Design review of the part built by this model. Coordinates are the model's own, in mm. A direction names the side the tool comes from. Coordinates: 2 decimals unless noted, no trailing zeros. Write each loop counter-clockwise with the first axis right and the second up, starting at its lowest first coordinate (ties: lowest second). Pieces come first, ordered by that corner, then holes. Notation, with made-up numbers: (33.5, 85) -> (56.5, 85) arc R15 cw to (56.5, 102) -> close; hole circle Ø1 at (22, 80). An arc over 180 degrees is marked (long way). Write item = value, one per line. Start each with the question number.
```python
from build123d import *

# Parameters (mm, degrees)
SKIZZE1_W                            = 51
SKIZZE1_H                            = 26
SKIZZE1_R                            = 9
AUFSATZ_LINEAR_AUSTRAGEN1_DEPTH      = 3
SKIZZE3_W                            = 51
SKIZZE3_H                            = 26
SKIZZE3_W_2                          = 47
SKIZZE3_H_2                          = 22
AUFSATZ_LINEAR_AUSTRAGEN3_DEPTH      = 10
AUFSATZ_LINEAR_AUSTRAGEN4_DEPTH      = 13
F_3_0_3_DURCHMESSER_BOHRUNG1_D       = 3
F_3_0_3_DURCHMESSER_BOHRUNG1_DEPTH   = 8
F_3_0_3_DURCHMESSER_BOHRUNG1_TIP     = 0.901290929
SCHNITT_LINEAR_AUSTRAGEN1_REACH      = 562.445
SKIZZE8_W                            = 13
SKIZZE8_H                            = 1
SKIZZE10_W                           = 35
SKIZZE10_H                           = 8
AUFSATZ_LINEAR_AUSTRAGEN5_DEPTH      = 10
F_1_5_1_5_DURCHMESSER_BOHRUNG1_D     = 1.5
F_1_5_1_5_DURCHMESSER_BOHRUNG1_DEPTH = 8
F_1_5_1_5_DURCHMESSER_BOHRUNG1_TIP   = 0.450645464


with BuildPart() as part:
    # Skizze1 → Aufsatz-Linear austragen1 (new body)
    with BuildSketch(Plane.XY):
        with Locations((526.252498469, 200.343199998)):
            Rectangle(SKIZZE1_W, SKIZZE1_H)
        with Locations((513.752498469, 200.343199998)):
            Circle(SKIZZE1_R, mode=Mode.SUBTRACT)
        with Locations((538.752498469, 200.343199998)):
            Circle(SKIZZE1_R, mode=Mode.SUBTRACT)
    extrude(amount=AUFSATZ_LINEAR_AUSTRAGEN1_DEPTH)

    # Skizze3 → Aufsatz-Linear austragen3 (add)
    with BuildSketch(Plane(origin=(0, 0, 0), x_dir=(-1, 0, 0), z_dir=(0, 0, -1))):
        with Locations((-526.252498469, 200.343199998)):
            Rectangle(SKIZZE3_W, SKIZZE3_H)
        with Locations((-526.252498469, 200.343199998)):
            Rectangle(SKIZZE3_W_2, SKIZZE3_H_2, mode=Mode.SUBTRACT)
    extrude(amount=AUFSATZ_LINEAR_AUSTRAGEN3_DEPTH)

    # Skizze4 → Aufsatz-Linear austragen4 (add)
    with BuildSketch(Plane(origin=(0, 0, -10), x_dir=(-1, 0, 0), z_dir=(0, 0, -1))):
        with BuildLine():
            Line((-496.752498469, 212.343199998), (-500.752498469, 212.343199998))
            Line((-500.752498469, 212.343199998), (-500.752498469, 204.343199998))
            Line((-500.752498469, 204.343199998), (-496.752498469, 204.343199998))
            ThreePointArc((-496.752498469, 204.343199998), (-492.752498469, 208.343199998), (-496.752498469, 212.343199998))
        make_face()
        with BuildLine():
            Line((-500.752498469, 196.343199998), (-496.752498469, 196.343199998))
            ThreePointArc((-496.752498469, 196.343199998), (-492.752498469, 192.343199998), (-496.752498469, 188.343199998))
            Line((-496.752498469, 188.343199998), (-500.752498469, 188.343199998))
            Line((-500.752498469, 188.343199998), (-500.752498469, 196.343199998))
        make_face()
        with BuildLine():
            Line((-551.752498469, 188.343199998), (-551.752498469, 196.343199998))
            Line((-551.752498469, 196.343199998), (-555.752498469, 196.343199998))
            ThreePointArc((-555.752498469, 196.343199998), (-559.752498469, 192.343199998), (-555.752498469, 188.343199998))
            Line((-555.752498469, 188.343199998), (-551.752498469, 188.343199998))
        make_face()
        with BuildLine():
            Line((-551.752498469, 204.343199998), (-555.752498469, 204.343199998))
            ThreePointArc((-555.752498469, 204.343199998), (-559.752498469, 208.343199998), (-555.752498469, 212.343199998))
            Line((-555.752498469, 212.343199998), (-551.752498469, 212.343199998))
            Line((-551.752498469, 212.343199998), (-551.752498469, 204.343199998))
        make_face()
    extrude(amount=-AUFSATZ_LINEAR_AUSTRAGEN4_DEPTH)

    # Ø3.0 (3) Durchmesser Bohrung1
    with Locations(Plane(origin=(0, 0, -10), x_dir=(-1, 0, 0), z_dir=(0, 0, -1))):
        with Locations((-555.752498469, 208.343199998), (-555.752498469, 192.343199998), (-496.752498469, 208.343199998), (-496.752498469, 192.343199998)):
            Hole(F_3_0_3_DURCHMESSER_BOHRUNG1_D / 2, depth=F_3_0_3_DURCHMESSER_BOHRUNG1_DEPTH)
            with Locations((0, 0, -(F_3_0_3_DURCHMESSER_BOHRUNG1_DEPTH + F_3_0_3_DURCHMESSER_BOHRUNG1_TIP / 2))):  # 118° drill point
                Cone(0, F_3_0_3_DURCHMESSER_BOHRUNG1_D / 2, F_3_0_3_DURCHMESSER_BOHRUNG1_TIP, mode=Mode.SUBTRACT)

    # Skizze8 → Schnitt-Linear austragen1 (cut, up to next)
    with BuildSketch(Plane.XZ.offset(-187.343199998), mode=Mode.PRIVATE) as schnitt_linear_austragen1_sk1:
        with Locations((526.252498469, -9.5)):
            Rectangle(SKIZZE8_W, SKIZZE8_H)
    schnitt_linear_austragen1_tool1 = extrude(schnitt_linear_austragen1_sk1.sketch, amount=-SCHNITT_LINEAR_AUSTRAGEN1_REACH, mode=Mode.PRIVATE) & part.part
    add(schnitt_linear_austragen1_tool1.solids().sort_by_distance((526.252498, 187.3432, -9.5))[0], mode=Mode.SUBTRACT)

    # Skizze10 → Aufsatz-Linear austragen5 (add)
    with BuildSketch(Plane.XZ.offset(-187.343199998)):
        with Locations((526.252498469, -3.5)):
            Rectangle(SKIZZE10_W, SKIZZE10_H)
    extrude(amount=AUFSATZ_LINEAR_AUSTRAGEN5_DEPTH)

    # Ø1.5 (1.5) Durchmesser Bohrung1
    with Locations(Plane(origin=(0, 177.343199998, 0), x_dir=(-1, 0, 0), z_dir=(0, -1, 0))):
        with Locations((-535.702498469, 3.5), (-516.802498469, 3.5)):
            Hole(F_1_5_1_5_DURCHMESSER_BOHRUNG1_D / 2, depth=F_1_5_1_5_DURCHMESSER_BOHRUNG1_DEPTH)
            with Locations((0, 0, -(F_1_5_1_5_DURCHMESSER_BOHRUNG1_DEPTH + F_1_5_1_5_DURCHMESSER_BOHRUNG1_TIP / 2))):  # 118° drill point
                Cone(0, F_1_5_1_5_DURCHMESSER_BOHRUNG1_D / 2, F_1_5_1_5_DURCHMESSER_BOHRUNG1_TIP, mode=Mode.SUBTRACT)


solid = part.part
```
(1) Take a section at D-D, the plane x = 527. State the section outline as (y, z) points.
(2) Take a section at A-A, the plane y = 194.5. State the section outline as (x, z) points, then the cut area to 3 significant figures.
(3) Take a section at B-B, the plane x = 512.5. State the section outline as (y, z) points, then the cut area to 3 significant figures.
(4) For faces 5 (the face through (526, 188, -9)), 6 (the face through (499, 212.343, -4)), 7 (the face through (527, 211.343, -5)), 8 (the face through (543.752, 182, -4)), 9 (the face through (499, 204.343, -4)), list the 3-axis set-ups (+Z, -Z, +X, -X, +Y, -Y) from which the entire face can be reached by the end or side of a thin tool; tool diameter is ignored.
(5) For line 1 (X direction, y = 182.5, z = -3.5); line 2 (Y direction, x = 531, z = -8); line 3 (Y direction, x = 532, z = -3.5), list the stretches that pass through material, from the lowest coordinate up.
(6) Take a section at C-C, the plane z = -6. Count the separate pieces of the cut face and the enclosed holes in it, then the cut area to 3 significant figures.
(7) For pin 1 Ø4 at (x, y) = (531.5, 204.5) entering from -Z; pin 2 Ø20.5 at (x, y) = (538.75, 200.34) entering from +Z; pin 3 Ø1 at (x, y) = (527, 188) entering from -Z; pin 4 Ø1 at (y, z) = (199, -1) entering from -X, all flat-tipped, find the tip position at first contact; note any pin that passes through.
(8) Mouldability with a two-part tool opening along Y and no side actions: class faces 1 (the face through (526, 182, -7.5)), 2 (the face through (516.906, 185.716, -3.421)), 3 (the face through (496.504, 192.421, -1.255)), 4 (the face through (499, 196.343, -4)) as pulls with the +Y half, pulls with the -Y half, needs draft (parallel to the pull), parting line crosses it, or undercut.
Report:
q1.outline = (177.34, -7.5) -> (187.34, -7.5) -> (187.34, -9) -> (189.34, -9) -> (189.34, 0) -> (211.34, 0) -> (211.34, -10) -> (213.34, -10) -> (213.34, 3) -> (187.34, 3) -> (187.34, 0.5) -> (177.34, 0.5) -> close
q2.outline = (493.38, -10) -> (502.75, -10) -> (502.75, 0) -> (506.91, 0) -> (506.91, 3) -> (493.38, 3) -> close; (520.6, 0) -> (531.91, 0) -> (531.91, 3) -> (520.6, 3) -> close; (545.6, 0) -> (549.75, 0) -> (549.75, -10) -> (559.12, -10) -> (559.12, 3) -> (545.6, 3) -> close
q2.area = 302 mm2
q3.outline = (177.34, -7.5) -> (187.34, -7.5) -> (187.34, -10) -> (189.34, -10) -> (189.34, 0) -> (191.43, 0) -> (191.43, 3) -> (187.34, 3) -> (187.34, 0.5) -> (177.34, 0.5) -> close; (209.26, 0) -> (211.34, 0) -> (211.34, -10) -> (213.34, -10) -> (213.34, 3) -> (209.26, 3) -> close
q3.area = 145 mm2
q4.face_5 = -Z, -Y
q4.face_6 = +Z, -Z, -X, +Y
q4.face_7 = -Z
q4.face_8 = +Z, -Z, +X, -Y
q4.face_9 = +Z, -Z, -X
q5.line_1 = 508.75 to 516.05, 517.55 to 534.95, 536.45 to 543.75
q5.line_2 = 187.34 to 189.34, 211.34 to 213.34
q5.line_3 = 177.34 to 189.34, 211.34 to 213.34
q6.separate_pieces = 1
q6.enclosed_holes = 5
q6.area = 842 mm2
q7.pin_1 = 0
q7.pin_2 = 3
q7.pin_3 = -9
q7.pin_4 = 500.75
q8.face_1 = needs draft
q8.face_2 = pulls with the -Y half
q8.face_3 = undercut
q8.face_4 = undercut
